from build123d import *

# Parameters (mm, degrees)
SKETCH1_R           = 12.25
BOSS_EXTRUDE1_DEPTH = 2.8
SKETCH2_R           = 16.5
BOSS_EXTRUDE2_DEPTH = 8
CHAMFER1_SIZE       = 3.5
SKETCH3_R           = 11.75
BOSS_EXTRUDE3_DEPTH = 29
SKETCH4_W           = 12
SKETCH4_H           = 26.533921206
BOSS_EXTRUDE4_DEPTH = 16


with BuildPart() as part:
    # Sketch1 → Boss-Extrude1 (new body)
    with BuildSketch(Plane(origin=(0, 0, 0), x_dir=(1, 0, 0), z_dir=(0, 1, 0))):
        Circle(SKETCH1_R)
    extrude(amount=BOSS_EXTRUDE1_DEPTH)

    # Sketch2 → Boss-Extrude2 (add)
    with BuildSketch(Plane.XZ):
        Circle(SKETCH2_R)
    extrude(amount=BOSS_EXTRUDE2_DEPTH)

    # Chamfer1
    chamfer1_edges = [part.edges().sort_by_distance(p)[0] for p in [
        (-16.5, 0, 0),
    ]]
    chamfer(chamfer1_edges, length=CHAMFER1_SIZE)

    # Sketch3 → Boss-Extrude3 (add)
    with BuildSketch(Plane.XZ.offset(8)):
        Circle(SKETCH3_R)
    extrude(amount=BOSS_EXTRUDE3_DEPTH)

    # Sketch4 → Boss-Extrude4 (add)
    with BuildSketch(Plane.XZ.offset(37)):
        with Locations((0, -0.455127293)):
            Rectangle(SKETCH4_W, SKETCH4_H)
    extrude(amount=BOSS_EXTRUDE4_DEPTH)


solid = part.part
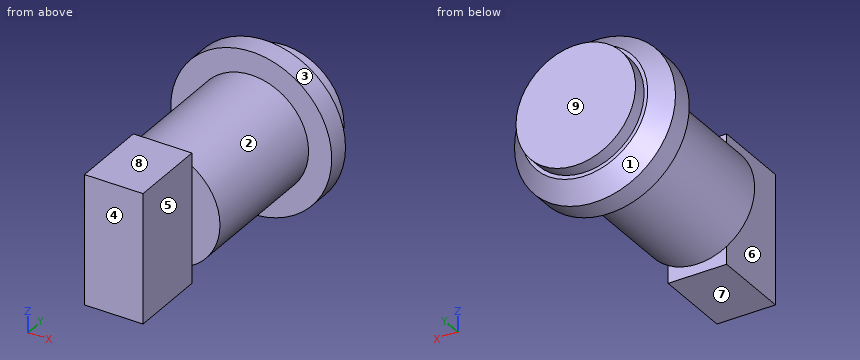
The model under review builds one solid part; all positions refer to its coordinate system, in mm. Face numbers are marked on the shaded views. A direction names the side the tool comes from. Give positions to 0.01 mm unless a question says otherwise; leave off trailing zeros. Write each loop counter-clockwise with the first axis right and the second up, starting at its lowest first coordinate (ties: lowest second). Pieces come first, ordered by that corner, then holes.
1. Add section C-C, the plane y = -31.5. Write out the cut boundary in (x, z).
2. For P1, Ø17.5, axis at y = -48, z = -5.5, coming from the +X side; P2, Ø10, axis at x = 3, y = -35.5, coming from the +Z side; P3, Ø10, axis at x = 4, y = -47, coming from the -Z side, all flat-tipped, find the tip position at first contact; note any pin that passes through.
3. Add section A-A, the plane x = 0. Write out the cut boundary in (y, z).
4. Add section B-B, the plane z = 0. Write out the cut boundary in (x, y).
5. Tool access review of the marked faces 5, 6, 7, 8 and 9: name each direction out of +Z, -Z, +X, -X, +Y, -Y from which nothing blocks a thin tool from reaching the whole face with its end or side.
6. Add section D-D, the plane y = -46.5. Write out the cut boundary in (x, z), plus the area to 3 significant figures.
7. Draft analysis for pull direction Y (two halves, no side actions). For the marked faces 1, 2, 3 and 4, state which applies: +Y half, -Y half, draft (parallel to the pull), parting line (faces both ways), or undercut.
8. Wall thickness on L1, parallel to X at y = -44.5, z = 0; L2, parallel to Y at x = 0.5, z = 12.5; L3, parallel to Z at x = -4, y = -38.5: over which ranges is each line inside the solid? List them lowest first.
Worked answers:
1. outline: circle Ø23.5 at (0, 0)
2. P1: stops at x = 6
2. P2: stops at z = 12.81
2. P3: stops at z = -13.72
3. outline: (-53, -13.72) - (-37, -13.72) - (-37, -11.75) - (-8, -11.75) - (-8, -16.5) - (-3.5, -16.5) - (0, -13) - (0, -12.25) - (2.8, -12.25) - (2.8, 12.25) - (0, 12.25) - (0, 13) - (-3.5, 16.5) - (-8, 16.5) - (-8, 11.75) - (-37, 11.75) - (-37, 12.81) - (-53, 12.81) - close
4. outline: (-16.5, -8) - (-11.75, -8) - (-11.75, -37) - (-6, -37) - (-6, -53) - (6, -53) - (6, -37) - (11.75, -37) - (11.75, -8) - (16.5, -8) - (16.5, -3.5) - (13, 0) - (12.25, 0) - (12.25, 2.8) - (-12.25, 2.8) - (-12.25, 0) - (-13, 0) - (-16.5, -3.5) - close
5. face 5: +Z, -Z, +X, -Y
5. face 6: +Z, -Z, -X, -Y
5. face 7: -Z, +X, -X, -Y
5. face 8: +Z, +X, -X, -Y
5. face 9: +Z, -Z, +X, -X, +Y
6. outline: (-6, -13.72) - (6, -13.72) - (6, 12.81) - (-6, 12.81) - close
6. area: 318 mm2
7. face 1: +Y half
7. face 2: undercut
7. face 3: draft
7. face 4: -Y half
8. L1: x = -6 to 6
8. L2: y = -53 to -37, -8 to 0
8. L3: z = -13.72 to 12.81
